Part model, mm, in its own coordinate system. A direction names the side the tool comes from. Coordinates: 2 decimals unless noted, no trailing zeros. Order: outer loops, then holes, each group sorted by start corner. A loop starts at its lowest first (then second) coordinate and runs counter-clockwise, first axis right, second up.
from build123d import *

# Parameters (mm, degrees)
BOSS_EXTRUDE1_DEPTH      = 6.100789
BOSS_EXTRUDE1_DEPTH_BACK = 8.899211
SKETCH2_R                = 1.51
CUT_EXTRUDE1_DEPTH       = 13.807078357
FILLET1_R                = 1
SKETCH3_W                = 24
SKETCH3_H                = 17
BOSS_EXTRUDE2_DEPTH      = 30
BOSS_EXTRUDE2_DEPTH_BACK = 3
SKETCH4_W                = 19.5
SKETCH4_H                = 15.5
CUT_EXTRUDE2_DEPTH       = 30
CUT_EXTRUDE6_DEPTH       = 3
FILLET2_R                = 1
SKETCH7_R                = 3.6
CUT_EXTRUDE7_DEPTH       = 25
CUT_EXTRUDE8_DEPTH       = 1
CUT_EXTRUDE8_DEPTH_BACK  = 25
CUT_EXTRUDE9_DEPTH       = 17.558078457
FILLET3_R                = 0.5


with BuildPart() as part:
    # Sketch1 → Boss-Extrude1 (new body, two sides)
    with BuildSketch(Plane.XY) as boss_extrude1_sk:
        with BuildLine():
            Line((4.558078357, 79.172152098), (3.25, 79.172152098))
            Line((3.25, 79.172152098), (3.25, 71.489520457))
            ThreePointArc((3.25, 71.489520457), (6.241751571, 66.453047962), (3.748333096, 61.152152098))
            Line((3.748333096, 61.152152098), (-3.748333096, 61.152152098))
            ThreePointArc((-3.748333096, 61.152152098), (-6.241751571, 66.453047962), (-3.25, 71.489520457))
            Line((-3.25, 71.489520457), (-3.25, 79.172152098))
            Line((-3.25, 79.172152098), (-4.558078357, 79.172152098))
            Line((-4.558078357, 79.172152098), (-4.558078357, 73.02746465))
            ThreePointArc((-4.558078357, 73.02746465), (-8.245549035, 66.39073565), (-4.947991632, 59.551896057))
            Line((-4.947991632, 59.551896057), (4.947991632, 59.551896057))
            ThreePointArc((4.947991632, 59.551896057), (8.245549035, 66.39073565), (4.558078357, 73.02746465))
            Line((4.558078357, 73.02746465), (4.558078357, 79.172152098))
        make_face()
    extrude(amount=BOSS_EXTRUDE1_DEPTH)
    extrude(boss_extrude1_sk.sketch, amount=-BOSS_EXTRUDE1_DEPTH_BACK)

    # Sketch2 → Cut-Extrude1 (cut, through all)
    with BuildSketch(Plane.ZY.offset(4.558078357)):
        with Locations((4.10078902, 76.662152098)):
            Circle(SKETCH2_R)
        with Locations((-3.39921098, 76.662152098)):
            Circle(SKETCH2_R)
    extrude(amount=-CUT_EXTRUDE1_DEPTH, mode=Mode.SUBTRACT)

    # Fillet1
    fillet1_edges = [part.edges().sort_by_distance(p)[0] for p in [
        (4.558078357, 73.02746465, -1.399211),
        (4.947991632, 59.551896057, -1.399211),
        (-4.947991632, 59.551896057, -1.399211),
        (-4.558078357, 73.02746465, -1.399211),
        (-3.904039179, 79.172152098, 6.100789),
        (3.904039179, 79.172152098, 6.100789),
        (3.904039179, 79.172152098, -8.899211),
        (-3.904039179, 79.172152098, -8.899211),
    ]]
    fillet(fillet1_edges, radius=FILLET1_R)

    # Sketch3 → Boss-Extrude2 (add, two sides)
    with BuildSketch(Plane(origin=(0, 0, -8.89921098), x_dir=(-1, 0, 0), z_dir=(0, 0, -1))) as boss_extrude2_sk:
        with Locations((0, 65.652152098)):
            Rectangle(SKETCH3_W, SKETCH3_H)
    extrude(amount=BOSS_EXTRUDE2_DEPTH)
    extrude(boss_extrude2_sk.sketch, amount=-BOSS_EXTRUDE2_DEPTH_BACK)

    # Sketch4 → Cut-Extrude2 (cut)
    with BuildSketch(Plane(origin=(0, 0, -38.89921098), x_dir=(-1, 0, 0), z_dir=(0, 0, -1))):
        with Locations((0, 66.402152098)):
            Rectangle(SKETCH4_W, SKETCH4_H)
    extrude(amount=-CUT_EXTRUDE2_DEPTH, mode=Mode.SUBTRACT)

    # Sketch6 → Cut-Extrude6 (cut)
    with BuildSketch(Plane(origin=(0, 0, -8.89921098), x_dir=(-1, 0, 0), z_dir=(0, 0, -1))):
        with BuildLine():
            Line((-3.25, 74.152152098), (-3.25, 71.489520457))
            ThreePointArc((-3.25, 71.489520457), (-6.241751571, 66.453047962), (-3.748333096, 61.152152098))
            Line((-3.748333096, 61.152152098), (3.748333096, 61.152152098))
            ThreePointArc((3.748333096, 61.152152098), (6.241751571, 66.453047962), (3.25, 71.489520457))
            Line((3.25, 71.489520457), (3.25, 74.152152098))
            Line((3.25, 74.152152098), (-3.25, 74.152152098))
        make_face()
    extrude(amount=-CUT_EXTRUDE6_DEPTH, mode=Mode.SUBTRACT)

    # Fillet2
    fillet2_edges = [part.edges().sort_by_distance(p)[0] for p in [
        (-4.663388941, 73.09814661, -5.89921098),
        (12, 74.152152098, -22.39921098),
        (-4.558078357, 74.152152098, -7.39921099),
        (4.558078357, 73.848493734, -5.89921098),
        (4.663388941, 73.09814661, -5.89921098),
        (8.247069912, 66.330586564, -5.89921098),
        (0, 59.551896057, -5.89921098),
        (-8.247069912, 66.330586564, -5.89921098),
        (-4.558078357, 73.848493734, -5.89921098),
        (12, 65.652152098, -5.89921098),
        (4.558078357, 74.152152098, -7.39921099),
        (-12, 74.152152098, -22.39921098),
        (-12, 65.652152098, -5.89921098),
        (-4.939958239, 59.610472754, -5.89921098),
        (4.939958239, 59.610472754, -5.89921098),
    ]]
    fillet(fillet2_edges, radius=FILLET2_R)

    # Sketch7 → Cut-Extrude7 (cut, through all)
    with BuildSketch(Plane.ZY.offset(12)):
        with Locations((-30.270250022, 66.152152098)):
            Circle(SKETCH7_R)
    extrude(amount=-CUT_EXTRUDE7_DEPTH, mode=Mode.SUBTRACT)

    # Sketch8 → Cut-Extrude8 (cut, two sides)
    with BuildSketch(Plane(origin=(12, 0, 0), x_dir=(0, 0, -1), z_dir=(1, 0, 0))) as cut_extrude8_sk:
        with BuildLine():
            Line((14.069083961, 74.152152098), (22.729337999, 74.152152098))
            ThreePointArc((22.729337999, 74.152152098), (18.39921098, 71.652152098), (14.069083961, 74.152152098))
        make_face()
    extrude(amount=CUT_EXTRUDE8_DEPTH, mode=Mode.SUBTRACT)
    extrude(cut_extrude8_sk.sketch, amount=-CUT_EXTRUDE8_DEPTH_BACK, mode=Mode.SUBTRACT)

    # Sketch9 → Cut-Extrude9 (cut, through all)
    with BuildSketch(Plane.ZY.offset(4.558078357)):
        with BuildLine():
            Line((-8.89921098, 78.172152098), (-8.89921098, 75.922152098))
            ThreePointArc((-8.89921098, 75.922152098), (-6.601113941, 76.874055059), (-5.64921098, 79.172152098))
            Line((-5.64921098, 79.172152098), (-7.89921098, 79.172152098))
            ThreePointArc((-7.89921098, 79.172152098), (-8.606317761, 78.879258879), (-8.89921098, 78.172152098))
        make_face()
    extrude(amount=-CUT_EXTRUDE9_DEPTH, mode=Mode.SUBTRACT)

    # Fillet3
    fillet3_edges = [part.edges().sort_by_distance(p)[0] for p in [
        (-3.904039179, 79.172152098, -5.64921098),
        (3.904039179, 79.172152098, -5.64921098),
        (-3.904039179, 75.922152098, -8.89921098),
        (3.904039179, 75.922152098, -8.89921098),
    ]]
    fillet(fillet3_edges, radius=FILLET3_R)


solid = part.part
Q1. Wall check: line 1 along X through (y, z) = (61.5, -9.5); line 2 along X through (y, z) = (76.5, -5.5); line 3 along Y through (x, z) = (-5, -21). Give the ranges that are in metal, low to high.
Results list:
line 1: x = -12 to -9.75, 9.75 to 12
line 2: x = -4.56 to -3.25, 3.25 to 4.56
line 3: y = 57.15 to 58.65
Q2. Cut at D-D on y = 67. Count the separate pieces of the cut face and the enclosed holes in it, and give its area (3 significant figures).
Results list:
separate pieces: 4
enclosed holes: 0
area: 187 mm2
Q3. Cut at B-B on x = -1.5. Write the cut outline in (y, z).
Results list:
outline: (57.15, -38.9) - (58.65, -38.9) - (58.65, -8.9) - (61.15, -8.9) - (61.15, 6.1) - (59.55, 6.1) - (59.55, -4.9) arc R1 cw to (58.55, -5.9) - (57.15, -5.9) - close
Q4. Mould opens along X. For faces 1 (the face through (-4.558, 76, 0)), 2 (the face through (11.715, 73.851, -10.301)), 3 (the face through (9, 74.152, -8)), 4 (the face through (0, 61.152, -2)) say: pulls with the +X half, pulls with the -X half, needs draft (parallel to the pull), parting line crosses it, or undercut.
Results list:
face 1: pulls with the -X half
face 2: pulls with the +X half
face 3: needs draft
face 4: undercut
Q5. Which spindle directions (+Z, -Z, +X, -X, +Y, -Y) get a long thin tool onto all of the face, cutting with end or side? Do faces 5 (the face through (4.558, 76, 0)), 6 (the face through (-3.913, 78.871, 5.816)), 7 (the face through (-9.75, 66, -24)). Say none if no direction does.
Results list:
face 5: +Z, +X, +Y
face 6: +Z, +X, -X, +Y
face 7: -Z, +Y
Q6. Cut at A-A on z = -2.5. Write the cut outline in (x, y).
Results list:
outline: (-5.24, 59.78) arc R1 ccw to (-4.6, 59.55) - (4.6, 59.55) arc R1 ccw to (5.24, 59.78) arc R8.25 ccw to (4.96, 72.75) arc R1 cw to (4.56, 73.54) - (4.56, 75.45) - (3.25, 75.45) - (3.25, 71.49) arc R6.25 cw to (3.75, 61.15) - (-3.75, 61.15) arc R6.25 cw to (-3.25, 71.49) - (-3.25, 75.45) - (-4.56, 75.45) - (-4.56, 73.54) arc R1 cw to (-4.96, 72.75) arc R8.25 ccw to start; (-4.56, 77.88) - (-3.25, 77.88) - (-3.25, 79.17) - (-4.56, 79.17) - close; (3.25, 77.88) - (4.56, 77.88) - (4.56, 79.17) - (3.25, 79.17) - close
Q7. Pin check, flat tips, straight feed: pin 1 Ø1 at (x, z) = (-10, -33) entering from +Y; pin 2 Ø9.5 at (y, z) = (66.15, -30.27) entering from -X; pin 3 Ø1 at (x, y) = (6.5, 71.5) entering from -Z; pin 4 Ø4 at (y, z) = (75, -1.5) entering from -X. Stop position of each tip, or through.
Results list:
pin 1: stops at y = 74.15
pin 2: stops at x = -12
pin 3: stops at z = -8.9
pin 4: stops at x = -4.72
Q8. Cut at C-C on z = -35.5. Write the cut outline in (x, y), and give its area (3 significant figures).
Results list:
outline: (-12, 57.15) - (12, 57.15) - (12, 73.15) arc R1 ccw to (11, 74.15) - (9.75, 74.15) - (9.75, 58.65) - (-9.75, 58.65) - (-9.75, 74.15) - (-11, 74.15) arc R1 ccw to (-12, 73.15) - close
area: 105 mm2
